Check sheet for the modelled part. Datum: model origin and axes. Units: mm. Face numbers are marked on the shaded views. A direction names the side the tool comes from. Give positions to 0.01 mm unless a question says otherwise; leave off trailing zeros. Write each loop counter-clockwise with the first axis right and the second up, starting at its lowest first coordinate (ties: lowest second). Pieces come first, ordered by that corner, then holes. Notation, with made-up numbers: M 54.5,72 L 87.5,72 A12 cw 87.5,94 Z; hole C 32,-29.75 d1. An arc over 180 degrees is marked long. One line per item, written item: value. Start each with the question number.
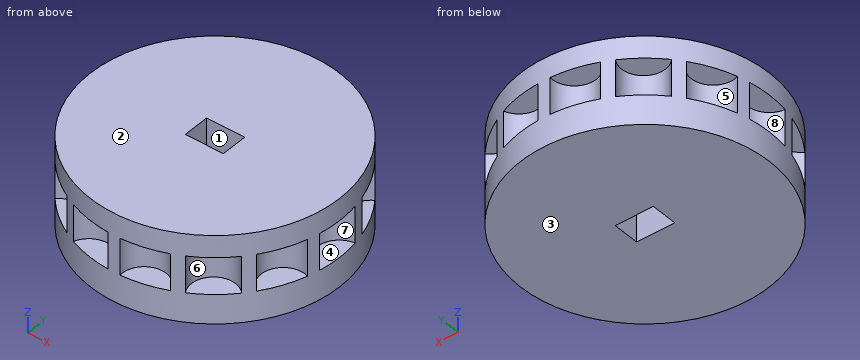
from build123d import *

# Parameters (mm, degrees)
F0_R      = 17
F1_DEPTH  = 4
F2_R      = 17
F3_DEPTH  = 5
F5_DEPTH  = 5
F6_COUNT  = 14
F7_R      = 17
F8_DEPTH  = 3
F9_W      = 5.2
F9_H      = 3.6
F10_DEPTH = 300


with BuildPart() as f1:
    # F0 (on Top) → F1 (new body)
    with BuildSketch(Plane.XY):
        Circle(F0_R)
    extrude(amount=F1_DEPTH)

    # F2 (on face) → F3 (join)
    with BuildSketch(Plane.XY.offset(4)):
        Circle(F2_R)
    extrude(amount=F3_DEPTH)

    # F6: F5 ×14 about axis
    f6_axis = Axis((0, 0, 9), (0, 0, 1))


with BuildPart() as f5:
    # F4 (on face) → F5 (new body)
    with BuildSketch(Plane.XY.offset(9)):
        with BuildLine():
            Line((19.066369161, -2.1748835579), (19.066369161, 2.1748835579))
            ThreePointArc((19.066369161, 2.1748835579), (18.1125082755, 2.7860949978), (17, 3))
            ThreePointArc((17, 3), (16.8675178144, 2.9970733175), (16.7352941176, 2.9882989803))
            ThreePointArc((16.7352941176, 2.9882989803), (16.9336942219, 1.5), (17, 0))
            ThreePointArc((17, 0), (16.9336942219, -1.5), (16.7352941176, -2.9882989803))
            ThreePointArc((16.7352941176, -2.9882989803), (16.8675178144, -2.9970733175), (17, -3))
            ThreePointArc((17, -3), (18.1125082755, -2.7860949978), (19.066369161, -2.1748835579))
        make_face()
        with BuildLine():
            ThreePointArc((17, 3), (18.1125082755, 2.7860949978), (19.066369161, 2.1748835579))
            Line((19.066369161, 2.1748835579), (19.066369161, 3))
            Line((19.066369161, 3), (17, 3))
        make_face()
        with BuildLine():
            ThreePointArc((17, 0), (16.9336942219, 1.5), (16.7352941176, 2.9882989803))
            ThreePointArc((16.7352941176, 2.9882989803), (14, 0), (16.7352941176, -2.9882989803))
            ThreePointArc((16.7352941176, -2.9882989803), (16.9336942219, -1.5), (17, 0))
        make_face()
    extrude(amount=-F5_DEPTH)


with BuildPart() as f1_1:
    add(f1.part)
    for i in range(1, F6_COUNT):
        add(f5.part.rotate(f6_axis, i * 360 / F6_COUNT), mode=Mode.SUBTRACT)

    # F6#seed: cut F5
    add(f5.part, mode=Mode.SUBTRACT)

    # F7 (on face) → F8 (join)
    with BuildSketch(Plane.XY.offset(9)):
        Circle(F7_R)
    extrude(amount=F8_DEPTH)

    # F9 (on face) → F10 (cut)
    with BuildSketch(Plane.XY.offset(12)):
        Rectangle(F9_W, F9_H)
    extrude(amount=-F10_DEPTH, mode=Mode.SUBTRACT)


solid = f1_1.part
1) Cross-section at B-B (x = 0). Record the boundary of the cut face in (y, z), plus the area to 3 significant figures.
2) Tool access check on the marked faces 1, 2, 3, 4 and 5. Record the directions out of +Z, -Z, +X, -X, +Y, -Y that give a thin tool (end or side, any length) a straight path to the whole face; none if there is none.
3) Cross-section at A-A (y = 0). Record the boundary of the cut face in (x, z).
4) Gauge pin test, flat ends, axial feed: pin 1 (6 mm diameter, centred on x = -8, z = 4, fed in from +Y); pin 2 (4 mm diameter, centred on y = -2.5, z = 10.5, fed in from +X); pin 3 (1.8 mm diameter, centred on y = 0.5, z = 5.5, fed in from +X). Record the tip position at first contact, or that the pin passes through.
5) Material ranges on L1, parallel to X at y = 0.5, z = 9.75; L2, parallel to Z at x = 2, y = 15.5; L3, parallel to Y at x = -8, z = 7.25, recorded low to high. Write a range as from..to.
6) Cross-section at C-C (x = 14.5). Record the boundary of the cut face in (y, z).
7) Draft check along X on the marked faces 6, 7 and 8. Enter one of: released by +X, released by -X, zero draft, split by the parting line, or undercut.
8) Cross-section at D-D (z = 1). Record the boundary of the cut face in (x, y), plus the area to 3 significant figures.
Data:
1. outline: M -17,0 L -1.8,0 L -1.8,12 L -17,12 Z; M 1.8,0 L 17,0 L 17,12 L 1.8,12 Z
1. area: 365 mm2
2. face 1: +Z, -Z
2. face 2: +Z, +X, -X, +Y, -Y
2. face 3: -Z, +X, -X, +Y, -Y
2. face 4: +X
2. face 5: none
3. outline: M -17,0 L -2.6,0 L -2.6,12 L -17,12 L -17,9 L -14,9 L -14,4 L -17,4 Z; M 2.6,0 L 17,0 L 17,4 L 14,4 L 14,9 L 17,9 L 17,12 L 2.6,12 Z
4. pin 1: stops at y = 16.25
4. pin 2: stops at x = 16.99
4. pin 3: stops at x = 14.35
5. L1: x = -16.99..-2.6, 2.6..16.99
5. L2: z = 0..4, 9..12
5. L3: y = -15..-14.79, -11.79..11.79, 14.79..15
6. outline: M -8.87,0 L 8.87,0 L 8.87,4 L 4.49,4 L 4.49,9 L 8.87,9 L 8.87,12 L -8.87,12 L -8.87,9 L -4.49,9 L -4.49,4 L -8.87,4 Z; hole M -1.66,4 L 1.66,4 L 1.66,9 L -1.66,9 Z
7. face 6: undercut
7. face 7: released by +X
7. face 8: released by -X
8. outline: C 0,0 d34; hole M -2.6,-1.8 L 2.6,-1.8 L 2.6,1.8 L -2.6,1.8 Z
8. area: 889 mm2
